Autodesk Inventor part; units mm, degrees
ref_plane "YZ Plane" through (0, 0, 0) normal (1, 0, 0) x (0, 1, 0)
ref_plane "XZ Plane" through (0, 0, 0) normal (0, 1, 0) x (-1, 0, 0)
ref_plane "XY Plane" through (0, 0, 0) normal (0, 0, 1) x (1, 0, 0)
sketch "Sketch1" plane through (0, 0, 0) normal (0, 0, 1) x (1, 0, 0)
  line L0 (-13.979, -55.38) -> (13.979, -55.38)
  line L1 (13.979, -55.38) -> (13.979, 55.38)
  line L2 (13.979, 55.38) -> (-13.979, 55.38)
  line L3 (-13.979, 55.38) -> (-13.979, -55.38)
  line L4 (-13.979, -55.38) -> (13.979, 55.38) construction
  line L5 (13.979, -55.38) -> (-13.979, 55.38) construction
  point P0 (0, 0)
  dimension "d0" = 27.958
  dimension "d1" = 110.76
extrude "Extrusion1" add sketch "Sketch1" along normal blind 30
sketch "Sketch2" plane through (0, 0, 0) normal (0, 0, -1) x (-1, 0, 0)
  line L0 (13.979, -55.38) -> (-13.979, -55.38) construction
  line L1 (0, -55.38) -> (0, -49.88) construction
  arc A0 (7.5, -49.88) -> (-7.5, -49.88) centre (0, -49.88) ccw
  line L2 (-7.5, -49.88) -> (-7.5, -55.38)
  line L3 (7.5, -49.88) -> (7.5, -55.38)
  line L4 (-13.979, 55.38) -> (13.979, 55.38) construction
  line L5 (0, 55.38) -> (0, 49.88) construction
  arc A1 (-5.5, 49.88) -> (5.5, 49.88) centre (0, 49.88) ccw
  line L6 (-5.5, 49.88) -> (-5.5, 55.38)
  line L7 (5.5, 49.88) -> (5.5, 55.38)
  line L8 (-5.5, 55.38) -> (5.5, 55.38)
  line L9 (-7.5, -55.38) -> (7.5, -55.38)
  point P0 (0, 0)
  dimension "d4" = 5.5
  dimension "d5" = 15
  dimension "d6" = 5.5
extrude "Extrusion2" cut sketch "Sketch2" against normal blind 10
sketch "Sketch3" plane through (0, 0, 10) normal (0, 0, -1) x (-1, 0, 0)
  arc A0 (-5.5, 49.88) -> (5.5, 49.88) centre (0, 49.88) ccw
  circle A1 centre (0, 49.88) radius 2.4
  arc A2 (7.5, -49.88) -> (-7.5, -49.88) centre (0, -49.88) ccw
  circle A3 centre (0, -49.88) radius 2.4
  point P0 (0, 0)
  dimension "d9" = 4.8
  dimension "d10" = 4.8
extrude "Extrusion3" cut sketch "Sketch3" against normal blind 10
sketch "Sketch4" plane through (0, 0, 30) normal (0, 0, 1) x (1, 0, 0)
  line L0 (-9.375, -39.5) -> (9.375, -39.5)
  line L1 (9.375, -39.5) -> (9.375, 39.5)
  line L2 (9.375, 39.5) -> (-9.375, 39.5)
  line L3 (-9.375, 39.5) -> (-9.375, -39.5)
  line L4 (-9.375, -39.5) -> (9.375, 39.5) construction
  line L5 (9.375, -39.5) -> (-9.375, 39.5) construction
  point P0 (0, 0)
  dimension "d13" = 18.75
  dimension "d14" = 79
extrude "Extrusion4" cut sketch "Sketch4" against normal blind 30
sketch "Sketch5" plane through (0, 0, 0) normal (0, 0, -1) x (-1, 0, 0)
  line L0 (9.375, -39.5) -> (-9.375, -39.5) construction
  line L1 (-9.375, -39.5) -> (-10.375, -39.5) construction
  line L2 (9.375, -39.5) -> (10.375, -39.5) construction
  line L3 (-10.375, -39.5) -> (10.375, -39.5)
  line L4 (10.375, -39.5) -> (10.375, -42)
  line L5 (10.375, -42) -> (-10.375, -42)
  line L6 (-10.375, -42) -> (-10.375, -39.5)
  line L7 (-9.375, -39.5) -> (-9.375, 39.5) construction
  line L8 (-9.375, 39.5) -> (-10.375, 39.5) construction
  line L9 (-9.375, 39.5) -> (9.375, 39.5) construction
  line L10 (9.375, 39.5) -> (10.375, 39.5) construction
  line L11 (-10.375, 39.5) -> (10.375, 39.5)
  line L12 (10.375, 39.5) -> (10.375, 42)
  line L13 (10.375, 42) -> (-10.375, 42)
  line L14 (-10.375, 42) -> (-10.375, 39.5)
  point P0 (0, 0)
  dimension "d17" = 1
  dimension "d18" = 1
  dimension "d19" = 2.5
  dimension "d20" = 1
  dimension "d21" = 1
  dimension "d22" = 2.5
extrude "Extrusion5" add sketch "Sketch5" along normal blind 125
sketch "Sketch6" plane through (-9.375, 39.5, 30) normal (0, -1, 0) x (1, 0, 0)
  line L0 (19.75, -30) -> (-1, -30) construction
  line L1 (19.75, -30) -> (19.75, -155) construction
  line L2 (19.75, -30) -> (19.75, -155) construction
  line L3 (19.75, -30) -> (19.75, -155)
  line L4 (19.75, -92.5) -> (18.75, -92.5)
  line L5 (18.75, -92.5) -> (18.75, -87.5)
  line L6 (18.75, -87.5) -> (19.75, -87.5)
  line L7 (19.75, -87.5) -> (19.75, -92.5)
  line L8 (-1, -30) -> (-1, -155)
  line L9 (-1, -92.5) -> (0, -92.5)
  line L10 (0, -92.5) -> (0, -87.5)
  line L11 (0, -87.5) -> (-1, -87.5)
  line L12 (-1, -87.5) -> (-1, -92.5)
  point P0 (9.375, -30)
  dimension "d25" = 1
  dimension "d26" = 5
  dimension "d27" = 1
  dimension "d28" = 5
extrude "Extrusion6" add sketch "Sketch6" along normal blind 80
properties part number "CyberDeckVerticalInsert4"
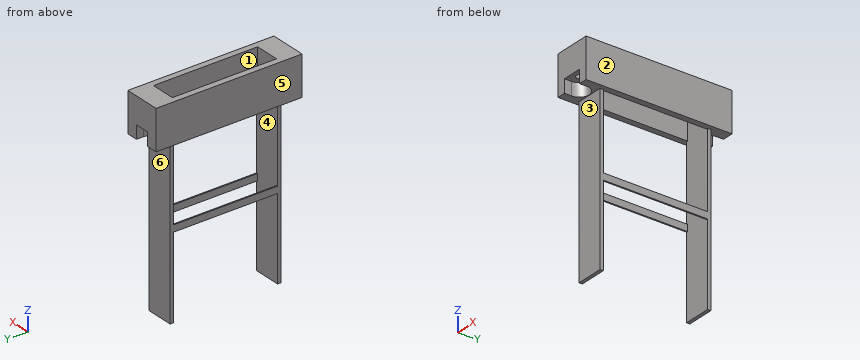
Geometry: final body of the model. Coordinates: model frame, mm. Face numbers are marked on the shaded views. A direction names the side the tool comes from. Give positions to 0.01 mm unless a question says otherwise; leave off trailing zeros. Loops run counter-clockwise (first coordinate to the right, second up) from the corner with the lowest first, then second, coordinate; pieces in that order, holes last. Notation, with made-up numbers: (36, 47) -> (68, 47) arc R32 cw to (68, 85) -> close; hole circle Ø10 at (-36, -20.75). An arc over 180 degrees is marked (long way). Return JSON: item names as keys, results as strings.
Item 1: Section B-B, the plane y = 18.5. Output: boundary loops of the cut face in (x, z) (3 decimals), plus the area to 3 significant figures.
Filled in:
{"outline": "(-13.979, 0) -> (-9.375, 0) -> (-9.375, 30) -> (-13.979, 30) -> close; (-10.375, -62.5) -> (-9.375, -62.5) -> (-9.375, -57.5) -> (-10.375, -57.5) -> close; (9.375, -62.5) -> (10.375, -62.5) -> (10.375, -57.5) -> (9.375, -57.5) -> close; (9.375, 0) -> (13.979, 0) -> (13.979, 30) -> (9.375, 30) -> close", "area": "286 mm^2"}
Item 2: Section A-A, the plane z = -42.5. Output: boundary loops of the cut face in (x, y) (3 decimals), plus the area to 3 significant figures.
Filled in:
{"outline": "(-10.375, -42) -> (10.375, -42) -> (10.375, -39.5) -> (-10.375, -39.5) -> close; (-10.375, 39.5) -> (10.375, 39.5) -> (10.375, 42) -> (-10.375, 42) -> close", "area": "104 mm^2"}
Item 3: Mould query, pull axis X, two halves, no side actions, for the marked faces 4, 5 and 6. Classes: released by +X, released by -X, zero draft, split by the parting line, or undercut.
Filled in:
{"face 4": "undercut", "face 5": "released by -X", "face 6": "zero draft"}
Item 4: Section C-C, the plane x = 0. Output: boundary loops of the cut face in (y, z), plus the area to 3 significant figures.
Filled in:
{"outline": "(-55.38, 10) -> (-52.28, 10) -> (-52.28, 20) -> (-47.48, 20) -> (-47.48, 10) -> (-42.38, 10) -> (-42.38, 0) -> (-42, 0) -> (-42, -125) -> (-39.5, -125) -> (-39.5, 30) -> (-55.38, 30) -> close; (39.5, -125) -> (42, -125) -> (42, 0) -> (44.38, 0) -> (44.38, 10) -> (47.48, 10) -> (47.48, 20) -> (52.28, 20) -> (52.28, 10) -> (55.38, 10) -> (55.38, 30) -> (39.5, 30) -> close", "area": "1,240 mm^2"}
Item 5: Line query: line 1 (Y direction, x = 0, z = 12); line 2 (Y direction, x = 7.5, z = -75.5); line 3 (X direction, y = -26.5, z = -60.5) (3 decimals). Output: solid intervals per line, ascending.
Filled in:
{"line 1": "-55.38 to -52.28, -47.48 to -39.5, 39.5 to 47.48, 52.28 to 55.38", "line 2": "-42 to -39.5, 39.5 to 42", "line 3": "-10.375 to -9.375, 9.375 to 10.375"}
Item 6: Pin query (flat end, axial travel): P1, Ø8, axis at x = -7.5, z = -22, coming from the +Y side; P2, Ø8, axis at y = 37, z = -75.5, coming from the +X side (3 decimals); P3, Ø5.5, axis at x = 0.5, y = -50, coming from the -Z side. Return the tip coordinate at first contact, or that it passes through.
Filled in:
{"P1": "y = 42", "P2": "x = 10.375", "P3": "z = 10"}
Item 7: Access query for the marked faces 1, 2 and 3. Directions: +Z, -Z, +X, -X, +Y, -Y. A direction counts if a zero-diameter tool reaches every point of the face in a straight line with its end or side. Return the directions, or none.
Filled in:
{"face 1": "+Z, -Z", "face 2": "+Z, -Z, +X, +Y, -Y", "face 3": "-Z, +X, -X, -Y"}
